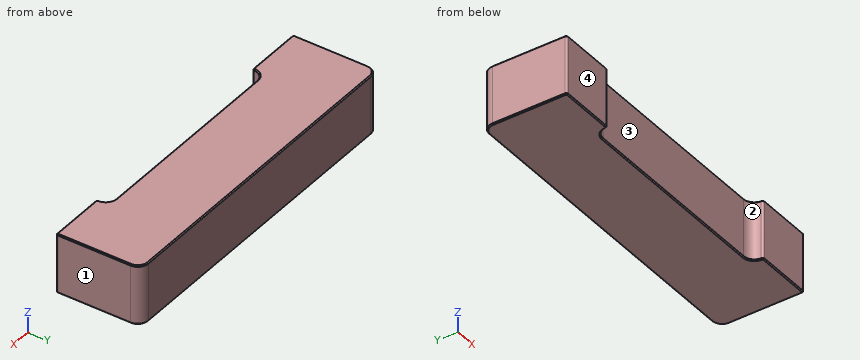
from build123d import *

# Parameters (mm, degrees)
F1_DEPTH = 11.3
F2_R     = 0.4
F3_SIZE  = 0.2


with BuildPart() as f1:
    # F0 (on Top) → F1 (new body)
    with BuildSketch(Plane.XY):
        with BuildLine():
            Line((-32, 6.05), (-32, -8.05))
            Line((-32, -8.05), (-21, -8.05))
            Line((-21, -8.05), (-21, -7.75))
            ThreePointArc((-21, -7.75), (-20.414214, -6.335786), (-19, -5.75))
            Line((-19, -5.75), (19, -5.75))
            ThreePointArc((19, -5.75), (20.414214, -6.335786), (21, -7.75))
            Line((21, -7.75), (21, -8.05))
            Line((21, -8.05), (32, -8.05))
            Line((32, -8.05), (32, 6.05))
            ThreePointArc((32, 6.05), (31.414214, 7.464214), (30, 8.05))
            Line((30, 8.05), (-30, 8.05))
            ThreePointArc((-30, 8.05), (-31.414214, 7.464214), (-32, 6.05))
        make_face()
    extrude(amount=F1_DEPTH)

    # F2
    f2_edges = [f1.edges().sort_by_distance(p)[0] for p in [
        (-32, -8.05, 5.65),
        (-21, -8.05, 5.65),
        (21, -8.05, 5.65),
        (32, -8.05, 5.65),
    ]]
    fillet(f2_edges, radius=F2_R)

    # F3
    f3_edges = [f1.edges().sort_by_distance(p)[0] for p in [
        (-32, -0.8, 0),
        (-31.882843, -7.932843, 0),
        (-31.414214, 7.464214, 0),
        (-26.498958, -8.05, 0),
        (0, 8.05, 0),
        (-21.121028, -7.938675, 0),
        (31.414214, 7.464214, 0),
        (-20.384437, -6.306624, 0),
        (32, -0.8, 0),
        (0, -5.75, 0),
        (31.882843, -7.932843, 0),
        (20.384437, -6.306624, 0),
        (26.498958, -8.05, 0),
        (21.121028, -7.938675, 0),
        (-32, -0.8, 11.3),
        (-31.882843, -7.932843, 11.3),
        (-31.414214, 7.464214, 11.3),
        (-26.498958, -8.05, 11.3),
        (0, 8.05, 11.3),
        (-21.121028, -7.938675, 11.3),
        (31.414214, 7.464214, 11.3),
        (-20.384437, -6.306624, 11.3),
        (32, -0.8, 11.3),
        (0, -5.75, 11.3),
        (31.882843, -7.932843, 11.3),
        (20.384437, -6.306624, 11.3),
        (26.498958, -8.05, 11.3),
        (21.121028, -7.938675, 11.3),
    ]]
    chamfer(f3_edges, length=F3_SIZE)


solid = f1.part
Can you work these out from the model? Positions are in its coordinate system, mm. Face numbers are marked on the shaded views. Coordinates: 2 decimals unless noted, no trailing zeros. Loops run counter-clockwise (first coordinate to the right, second up) from the corner with the lowest first, then second, coordinate; pieces in that order, holes last. Notation, with made-up numbers: (30.25, -29.75) - (74.25, -29.75) arc R10 cw to (74.25, -13.75) - close; hole circle Ø7 at (-11, -39.75). An arc over 180 degrees is marked (long way). Answer as a JSON object with one key per item and string values. Group by question number.
Item 1: If we mould it in two halves opening along X, with no side actions, what happens to the marked faces 1, 2, 3 and 4? For each: released by +X, released by -X, zero draft, split by the parting line, or undercut.
Item 2: If I drill on L1, parallel to Y at x = -16, z = 6.75; L2, parallel to X at y = -7, z = 7.5; L3, parallel to X at y = 7, z = 2, over which ranges is the centre line in solid material (lowest first)? Write a range as from..to.
Item 3: For pin 1 (3.5 mm diameter, centred on x = 0.5, z = 5, fed in from -Y); pin 2 (3 mm diameter, centred on x = 18, z = 6, fed in from -Y), each with a flat end and sliding along its axis, tell me the tip position at first contact or that it passes through.
Item 4: If we section it at A-A (x = 14): List the corners of the cut face in (y, z) for me.
Returned:
{
 "1": {"face 1": "released by +X", "face 2": "undercut", "face 3": "undercut", "face 4": "zero draft"},
 "2": {"L1": "y = -5.75..8.05", "L2": "x = -32..-20.85, 20.85..32", "L3": "x = -31.76..31.76"},
 "3": {"pin 1": "stops at y = -5.75", "pin 2": "stops at y = -5.81"},
 "4": {"outline": "(-5.75, 0.2) - (-5.55, 0) - (7.85, 0) - (8.05, 0.2) - (8.05, 11.1) - (7.85, 11.3) - (-5.55, 11.3) - (-5.75, 11.1) - close"}
}
